```python
from build123d import *

# Parameters (mm, degrees)
CYLINDER016_R             = 1.75
CYLINDER016_DEPTH         = 70
CYLINDER016_ROLL_ANGLE    = -90
CYLINDER026_R             = 1.75
CYLINDER026_DEPTH         = 24.5
CYLINDER026_PITCH_ANGLE   = 90
CYLINDER027_R             = 3
CYLINDER027_DEPTH         = 21.5
CYLINDER027_PITCH_ANGLE   = 90
FUSION007_PITCH_ANGLE     = -90
FUSION007_PLACEMENT_ANGLE = -180
FUSION008_PITCH_ANGLE     = -90
FUSION008_PLACEMENT_ANGLE = -180
FUSION005_PITCH_ANGLE     = -90
FUSION005_PLACEMENT_ANGLE = -180
FUSION006_PITCH_ANGLE     = -90
FUSION006_PLACEMENT_ANGLE = -180
BOX021_W                  = 37
BOX021_H                  = 41
BOX021_DEPTH              = 25
BOX021_PITCH_ANGLE        = -90
BOX021_PLACEMENT_ANGLE    = -180
FUSION012_PITCH_ANGLE     = -90
FUSION012_PLACEMENT_ANGLE = -90
BOX007_W                  = 68
BOX007_H                  = 10.5
BOX007_DEPTH              = 29
CHAMFER_SIZE              = 12
BOX057_W                  = 12
BOX057_H                  = 16
BOX057_DEPTH              = 10
PAD005_DEPTH              = 2.5
CHAMFER009_SIZE           = 4


with BuildPart() as cylinder016:
    # Cylinder016 → Cylinder016 (new body)
    with BuildSketch(Plane.XY):
        Circle(CYLINDER016_R)
    extrude(amount=CYLINDER016_DEPTH)


with BuildPart() as cylinder016_1:
    # Cylinder016 roll: moved
    add(cylinder016.part.rotate(Axis((0, 0, 0), (1, 0, 0)), CYLINDER016_ROLL_ANGLE))


with BuildPart() as cylinder016_2:
    # Cylinder016 placement: moved
    add(cylinder016_1.part.moved(Location((-40.5, -5, -149.5))))


with BuildPart() as joint_d010:
    # Cylinder026 → Cylinder026 (new body)
    with BuildSketch(Plane.XY):
        Circle(CYLINDER026_R)
    extrude(amount=CYLINDER026_DEPTH)


with BuildPart() as joint_d010_1:
    # Cylinder026 pitch: moved
    add(joint_d010.part.rotate(Axis((0, 0, 0), (0, 1, 0)), CYLINDER026_PITCH_ANGLE))


with BuildPart() as joint_d010_2:
    # Cylinder026 placement: moved
    add(joint_d010_1.part.moved(Location((16, -24.5, 7))))


with BuildPart() as joint_d011:
    # Cylinder027 → Cylinder027 (new body)
    with BuildSketch(Plane.XY):
        Circle(CYLINDER027_R)
    extrude(amount=CYLINDER027_DEPTH)


with BuildPart() as joint_d011_1:
    # Cylinder027 pitch: moved
    add(joint_d011.part.rotate(Axis((0, 0, 0), (0, 1, 0)), CYLINDER027_PITCH_ANGLE))


with BuildPart() as joint_d011_2:
    # Cylinder027 placement: moved
    add(joint_d011_1.part.moved(Location((37, -24.5, 7))))


with BuildPart() as fusion007:
    # Fusion007 base: copy of Joint-D011
    add(joint_d011_2.part)

    # Fusion007: union Joint-D010
    add(joint_d010_2.part)


with BuildPart() as fusion007_1:
    # Fusion007 pitch: moved
    add(fusion007.part.rotate(Axis((0, 0, 0), (0, 1, 0)), FUSION007_PITCH_ANGLE))


with BuildPart() as fusion007_2:
    # Fusion007 placement: moved
    add(fusion007_1.part.moved(Location((-12, -39.5, 0))).rotate(Axis((-12, -39.5, 0), (0, 0, 1)), FUSION007_PLACEMENT_ANGLE))


with BuildPart() as fusion008:
    # Fusion008 base: copy of Joint-D011
    add(joint_d011_2.part)

    # Fusion008: union Joint-D010
    add(joint_d010_2.part)


with BuildPart() as fusion008_1:
    # Fusion008 pitch: moved
    add(fusion008.part.rotate(Axis((0, 0, 0), (0, 1, 0)), FUSION008_PITCH_ANGLE))


with BuildPart() as fusion008_2:
    # Fusion008 placement: moved
    add(fusion008_1.part.moved(Location((-2, -39.5, 0))).rotate(Axis((-2, -39.5, 0), (0, 0, 1)), FUSION008_PLACEMENT_ANGLE))


with BuildPart() as fusion005:
    # Fusion005 base: copy of Joint-D011
    add(joint_d011_2.part)

    # Fusion005: union Joint-D010
    add(joint_d010_2.part)


with BuildPart() as fusion005_1:
    # Fusion005 pitch: moved
    add(fusion005.part.rotate(Axis((0, 0, 0), (0, 1, 0)), FUSION005_PITCH_ANGLE))


with BuildPart() as fusion005_2:
    # Fusion005 placement: moved
    add(fusion005_1.part.moved(Location((-12, 9.5, 0))).rotate(Axis((-12, 9.5, 0), (0, 0, 1)), FUSION005_PLACEMENT_ANGLE))


with BuildPart() as fusion006:
    # Fusion006 base: copy of Joint-D011
    add(joint_d011_2.part)

    # Fusion006: union Joint-D010
    add(joint_d010_2.part)


with BuildPart() as fusion006_1:
    # Fusion006 pitch: moved
    add(fusion006.part.rotate(Axis((0, 0, 0), (0, 1, 0)), FUSION006_PITCH_ANGLE))


with BuildPart() as fusion006_2:
    # Fusion006 placement: moved
    add(fusion006_1.part.moved(Location((-2, 9.5, 0))).rotate(Axis((-2, 9.5, 0), (0, 0, 1)), FUSION006_PLACEMENT_ANGLE))


with BuildPart() as fusion012:
    # Box021 → Box021 (new body)
    with BuildSketch(Plane.XY):
        with Locations((18.5, 20.5)):
            Rectangle(BOX021_W, BOX021_H)
    extrude(amount=BOX021_DEPTH)


with BuildPart() as fusion012_1:
    # Box021 pitch: moved
    add(fusion012.part.rotate(Axis((0, 0, 0), (0, 1, 0)), BOX021_PITCH_ANGLE))


with BuildPart() as fusion012_2:
    # Box021 placement: moved
    add(fusion012_1.part.moved(Location((-10, 30, -1))).rotate(Axis((-10, 30, -1), (0, 0, 1)), BOX021_PLACEMENT_ANGLE))

    # Fusion012: union Fusion007, Fusion008, Fusion005, Fusion006
    add(fusion007_2.part)
    add(fusion008_2.part)
    add(fusion005_2.part)
    add(fusion006_2.part)


with BuildPart() as fusion012_3:
    # Fusion012 pitch: moved
    add(fusion012_2.part.rotate(Axis((0, 0, 0), (0, 1, 0)), FUSION012_PITCH_ANGLE))


with BuildPart() as fusion012_4:
    # Fusion012 placement: moved
    add(fusion012_3.part.moved(Location((-16.5, -5, -134))).rotate(Axis((-16.5, -5, -134), (0, 0, 1)), FUSION012_PLACEMENT_ANGLE))


with BuildPart() as chamfer_body:
    # Box007 → Box007 (new body)
    with BuildSketch(Plane(origin=(-35, 18, -153.5), x_dir=(1, 0, 0), z_dir=(0, 0, 1))):
        with Locations((34, 5.25)):
            Rectangle(BOX007_W, BOX007_H)
    extrude(amount=BOX007_DEPTH)

    # Chamfer
    chamfer_edges = [chamfer_body.edges().sort_by_distance(p)[0] for p in [
        (33, 23.25, -124.5),
    ]]
    chamfer(chamfer_edges, length=CHAMFER_SIZE)


with BuildPart() as cube060:
    # Box057 → Box057 (new body)
    with BuildSketch(Plane(origin=(-47, 24.5, -155), x_dir=(1, 0, 0), z_dir=(0, 0, 1))):
        with Locations((6, 8)):
            Rectangle(BOX057_W, BOX057_H)
    extrude(amount=BOX057_DEPTH)


with BuildPart() as clone_of_chamfer009:
    # Sketch007 → Pad005 (new body)
    with BuildSketch(Plane(origin=(0, 0, -155), x_dir=(1, 0, 0), z_dir=(0, 0, -1))):
        Polygon((-47, -17.5), (-47, -3), (-30.5, -3), (-19, -9.5), (5, -9.5), (16.5, -3), (33, -3), (33, -59.5), (16.5, -59.5), (5, -53), (-19, -53), (-30.5, -59.5), (-47, -59.5), (-47, -47.5), (-36, -47.5), (-36, -17.5), align=None)
    extrude(amount=-PAD005_DEPTH)

    # Fusion: union Chamfer body, Cube060
    add(chamfer_body.part)
    add(cube060.part)

    # Cut083: cut Fusion012
    add(fusion012_4.part, mode=Mode.SUBTRACT)

    # Cut084: cut Cylinder016
    add(cylinder016_2.part, mode=Mode.SUBTRACT)

    # Chamfer009
    chamfer009_edges = [clone_of_chamfer009.edges().sort_by_distance(p)[0] for p in [
        (-47, 32.5, -145),
    ]]
    chamfer(chamfer009_edges, length=CHAMFER009_SIZE)


with BuildPart() as clone_of_chamfer009_1:
    # Chamfer009 placement: moved
    add(clone_of_chamfer009.part.moved(Location((0, 0, 94))))


with BuildPart() as clone_of_chamfer009_2:
    # Clone015 placement: moved
    add(clone_of_chamfer009_1.part.moved(Location((0, 0, -70.710678))))


solid = clone_of_chamfer009_2.part
```
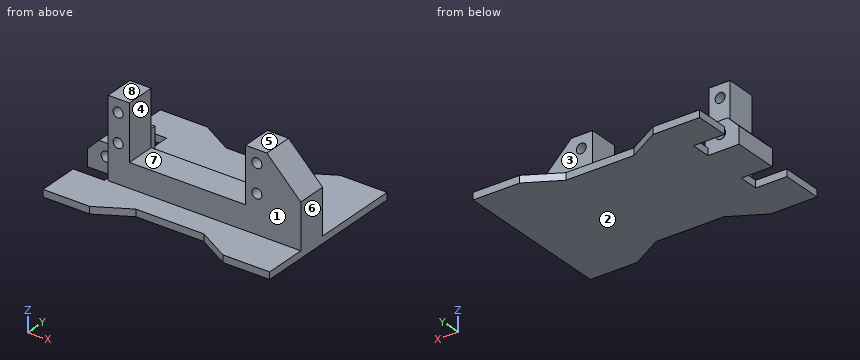
Check sheet for the modelled part. Datum: model origin and axes. Units: mm. Face numbers are marked on the shaded views. A direction names the side the tool comes from. Round coordinates to 2 decimals unless told otherwise and drop trailing zeros. Order: outer loops, then holes, each group sorted by start corner. A loop starts at its lowest first (then second) coordinate and runs counter-clockwise, first axis right, second up. Notation, with made-up numbers: (44, -37) - (50, -37) arc R19 cw to (50, -22) - close; hole circle Ø10 at (54, 63). An arc over 180 degrees is marked (long way). Answer as CSV lines item,"result". Start each with the question number.
1) Section check B-B (x = -40.5). Record the cut outline in (y, z).
2) Section check D-D (x = -2). Record the cut outline in (y, z), then the cut area to 3 significant figures.
3) Section check C-C (y = 34). Record the cut outline in (x, z).
4) Depth check by flat-ended pin: pin 1 (3 mm diameter, centred on x = -25.5, z = -112, fed in from +Y); pin 2 (3 mm diameter, centred on x = -9, y = 26.5, fed in from +Z); pin 3 (4 mm diameter, centred on x = -37.5, y = 30, fed in from +Z); pin 4 (1.2 mm diameter, centred on x = -7, z = -130.5, fed in from +Y). Enter the tip coordinate at first touch or a pass-through.
5) Tool access check on the marked faces 1, 2, 3, 4 and 5. Record the directions out of +Z, -Z, +X, -X, +Y, -Y that give a thin tool (end or side, any length) a straight path to the whole face; none if there is none.
6) Draft check along X on the marked faces 6, 7 and 8. Enter one of: +X half, -X half, draft (parallel to the pull), parting line (faces both ways), or undercut.
7) Scan lines: probe 1 along Z at (x, y) = (-31, 21); probe 2 along Z at (x, y) = (-31.5, 21); probe 3 along Z at (x, y) = (-40.5, 31.5). Record each from-to range of solid material in increasing order.
8) Section check A-A (x = 17.5). Record the cut outline in (y, z).
Determined:
1,outline,"(3, -131.71) - (17.5, -131.71) - (17.5, -129.21) - (3, -129.21) - close; (24.5, -131.71) - (40.5, -131.71) - (40.5, -127.96) - (24.5, -127.96) - close; (24.5, -124.46) - (40.5, -124.46) - (40.5, -121.71) - (24.5, -121.71) - close; (47.5, -131.71) - (59.5, -131.71) - (59.5, -129.21) - (47.5, -129.21) - close"
2,outline,"(9.5, -131.71) - (53, -131.71) - (53, -129.21) - (28.5, -129.21) - (28.5, -120.71) - (18, -120.71) - (18, -129.21) - (9.5, -129.21) - close"
2,area,"198 mm^2"
3,outline,"(-47, -131.71) - (33, -131.71) - (33, -129.21) - (-35, -129.21) - (-35, -121.71) - (-43, -121.71) - (-47, -125.71) - close; hole circle Ø3.5 at (-40.5, -126.21)"
4,pin 1,"through"
4,pin 2,"z = -120.71"
4,pin 3,"z = -121.71"
4,pin 4,"y = 53"
5,face 1,"+Z, +X, -X, -Y"
5,face 2,"-Z, +X, -X, +Y, -Y"
5,face 3,"+Z, +X, +Y"
5,face 4,"+Z, +Y, -Y"
5,face 5,"+Z, +X, -X, +Y, -Y"
6,face 6,"+X half"
6,face 7,"undercut"
6,face 8,"draft"
7,probe 1,"-131.71 to -117.39, -114.03 to -107.39, -104.03 to -101.21"
7,probe 2,"-131.71 to -117.46, -113.96 to -107.46, -103.96 to -101.21"
7,probe 3,"-131.71 to -127.96, -124.46 to -121.71"
8,outline,"(3, -131.71) - (59.5, -131.71) - (59.5, -129.21) - (28.5, -129.21) - (28.5, -117.46) - (18, -117.46) - (18, -129.21) - (3, -129.21) - close; (18, -113.96) - (28.5, -113.96) - (28.5, -107.46) - (18, -107.46) - close; (18, -103.96) - (28.5, -103.96) - (28.5, -101.21) - (18, -101.21) - close"
